from build123d import *

# Parameters (mm, degrees)
ESBO_O1_W                = 200
ESBO_O1_H                = 150
ESBO_O1_R                = 4.015931703
RESSALTO_EXTRUS_O1_DEPTH = 100
ESBO_O2_W                = 187.670035944
ESBO_O2_H                = 140.530338622
CORTE_EXTRUS_O2_DEPTH    = 80
ESBO_O3_W                = 25.727524856
ESBO_O3_H                = 8.994175356
CORTE_EXTRUS_O3_DEPTH    = 103
ESBO_O4_W                = 11.504177781
ESBO_O4_H                = 7.948341013
CORTE_EXTRUS_O4_DEPTH    = 114
ESBO_O5_W                = 71.332240634
ESBO_O5_H                = 44.178578037
CORTE_EXTRUS_O5_DEPTH    = 114


with BuildPart() as part:
    # Esboço1 → Ressalto-extrusão1 (new body)
    with BuildSketch(Plane.XY):
        Rectangle(ESBO_O1_W, ESBO_O1_H)
        with Locations((-87.500730847, 65.625548135)):
            Circle(ESBO_O1_R, mode=Mode.SUBTRACT)
        with Locations(Location((-87.500730847, -65.625548135, 0), (0, 0, 180))):
            Circle(ESBO_O1_R, mode=Mode.SUBTRACT)
        with Locations(Location((87.500730847, 65.625548135, 0), (0, 0, 180))):
            Circle(ESBO_O1_R, mode=Mode.SUBTRACT)
        with Locations((87.500730847, -65.625548135)):
            Circle(ESBO_O1_R, mode=Mode.SUBTRACT)
    extrude(amount=RESSALTO_EXTRUS_O1_DEPTH)

    # Esboço2 → Corte-extrusão2 (cut)
    with BuildSketch(Plane.XY):
        Rectangle(ESBO_O2_W, ESBO_O2_H)
    extrude(amount=CORTE_EXTRUS_O2_DEPTH, mode=Mode.SUBTRACT)

    # Esboço3 → Corte-extrusão3 (cut)
    with BuildSketch(Plane(origin=(0, 0, 0), x_dir=(0, 0, -1), z_dir=(1, 0, 0))):
        with Locations((-20.821221809, -65.887563657)):
            Rectangle(ESBO_O3_W, ESBO_O3_H)
    extrude(amount=-CORTE_EXTRUS_O3_DEPTH, mode=Mode.SUBTRACT)

    # Esboço4 → Corte-extrusão4 (cut)
    with BuildSketch(Plane(origin=(0, 0, 0), x_dir=(0, 0, -1), z_dir=(1, 0, 0))):
        with Locations((-86.08128486, -65.992147092)):
            Rectangle(ESBO_O4_W, ESBO_O4_H)
        with Locations((-14.337048878, -65.992147092)):
            Rectangle(ESBO_O4_W, ESBO_O4_H)
    extrude(amount=CORTE_EXTRUS_O4_DEPTH, mode=Mode.SUBTRACT)

    # Esboço5 → Corte-extrusão5 (cut)
    with BuildSketch(Plane(origin=(0, 75, 0), x_dir=(1, 0, 0), z_dir=(0, 1, 0))):
        with Locations((1.831794699, -49.568989483)):
            Rectangle(ESBO_O5_W, ESBO_O5_H)
    extrude(amount=-CORTE_EXTRUS_O5_DEPTH, mode=Mode.SUBTRACT)


solid = part.part
Could you check a few things on this model? Use its own coordinates, in mm. A direction names the side the tool comes from. Round coordinates to 2 decimals unless told otherwise and drop trailing zeros. Write each loop counter-clockwise with the first axis right and the second up, starting at its lowest first coordinate (ties: lowest second). Pieces come first, ordered by that corner, then holes. Notation, with made-up numbers: (89.25, 24) -> (99.25, 24) arc R23 cw to (99.25, 61) -> close; hole circle Ø7 at (70, 62.5). An arc over 180 degrees is marked (long way). Use a Markdown table: item, result.
1. If we section it at A-A (x = 30): List the corners of the cut face in (y, z) for me, then the cut area to 3 significant figures.
Answer key:
| item | result |
|---|---|
| outline | (-75, 0) -> (-70.27, 0) -> (-70.27, 80) -> (70.27, 80) -> (70.27, 71.66) -> (75, 71.66) -> (75, 100) -> (-75, 100) -> close; (70.27, 0) -> (75, 0) -> (75, 27.48) -> (70.27, 27.48) -> close; hole (-69.97, 80.33) -> (-62.02, 80.33) -> (-62.02, 91.83) -> (-69.97, 91.83) -> close |
| area | 3,460 mm^2 |
2. If we section it at B-B (x = -26.5): List the corners of the cut face in (y, z) for me, then the cut area to 3 significant figures.
Answer key:
| item | result |
|---|---|
| outline | (-75, 0) -> (-70.27, 0) -> (-70.27, 7.96) -> (-70.38, 7.96) -> (-70.38, 33.68) -> (-70.27, 33.68) -> (-70.27, 80) -> (70.27, 80) -> (70.27, 71.66) -> (75, 71.66) -> (75, 100) -> (-75, 100) -> close; (70.27, 0) -> (75, 0) -> (75, 27.48) -> (70.27, 27.48) -> close |
| area | 3,550 mm^2 |
3. For pin 1 Ø10 at (x, z) = (4, 38) entering from +Y; pin 2 Ø1.5 at (x, y) = (40, 53) entering from -Z, each with a flat end and sliding along its axis, tell me the tip position at first contact or that it passes through.
Answer key:
| item | result |
|---|---|
| pin 1 | stops at y = -70.27 |
| pin 2 | stops at z = 80 |
4. If we section it at C-C (z = 88.5): List the corners of the cut face in (x, y) for me, then the cut area to 3 significant figures.
Answer key:
| item | result |
|---|---|
| outline | (-100, -75) -> (100, -75) -> (100, -69.97) -> (0, -69.97) -> (0, -62.02) -> (85.74, -62.02) arc R4.02 cw to (89.27, -62.02) -> (100, -62.02) -> (100, 75) -> (-100, 75) -> close; hole circle Ø8.03 at (-87.5, -65.63); hole circle Ø8.03 at (-87.5, 65.63); hole circle Ø8.03 at (87.5, 65.63) |
| area | 29,100 mm^2 |
5. Please list where these lines run through material, in increasing order: probe 1 along X at (y, z) = (14, 58.5); probe 2 along Y at (x, z) = (70.5, 38); probe 3 along Z at (x, y) = (-86, 51.5).
Answer key:
| item | result |
|---|---|
| probe 1 | x = -100 to -93.84, 93.84 to 100 |
| probe 2 | y = -75 to -70.27, 70.27 to 75 |
| probe 3 | z = 80 to 100 |
6. We'd pull the mould along Y, two halves only. Please class faces 1 (the face through (97, -69.966, 14)), 2 (the face through (-1, 75, 27)), 3 (the face through (-8, -72, 0)): +Y half, -Y half, draft (parallel to the pull), parting line (faces both ways), or undercut.
Answer key:
| item | result |
|---|---|
| face 1 | undercut |
| face 2 | +Y half |
| face 3 | draft |
7. Which directions (+Z, -Z, +X, -X, +Y, -Y) give clear straight access to the entire face, cutting with the end or side of a thin tool? Please do faces 4 (the face through (-97, -61.39, 21)), 5 (the face through (1, 73, 27.48)), 6 (the face through (93.835, -1, 39)).
Answer key:
| item | result |
|---|---|
| face 4 | -X |
| face 5 | +Y |
| face 6 | -Z |
8. If we section it at D-D (y = -56.5): List the corners of the cut face in (x, z) for me, then the cut area to 3 significant figures.
Answer key:
| item | result |
|---|---|
| outline | (-100, 0) -> (-93.84, 0) -> (-93.84, 80) -> (93.84, 80) -> (93.84, 0) -> (100, 0) -> (100, 100) -> (-100, 100) -> close |
| area | 4,990 mm^2 |
